```python
from build123d import *

# Parameters (mm, degrees)
SKETCH1_W                = 6.4
SKETCH1_H                = 22.2
SKETCH1_W_2              = 0.8
SKETCH1_H_2              = 2
BOSS_EXTRUDE1_DEPTH      = 13.7
BOSS_EXTRUDE2_DEPTH      = 3
SKETCH2_W                = 9
SKETCH2_H                = 2.5
CUT_EXTRUDE1_DEPTH       = 27.513015672
SKETCH2_3_W              = 2.5
SKETCH2_3_H              = 3
CUT_EXTRUDE2_DEPTH       = 0.2
CUT_EXTRUDE3_DEPTH       = 0.3
BOSS_EXTRUDE3_DEPTH      = 6.5
BOSS_EXTRUDE3_DEPTH_BACK = 6.5
SKETCH4_W                = 0.7
SKETCH4_H                = 3.8
BOSS_EXTRUDE4_DEPTH      = 4
BOSS_EXTRUDE4_DEPTH_BACK = 4
SKETCH4_3_W              = 0.3
SKETCH4_3_H              = 6.2
SKETCH7_R                = 0.25
SKETCH7_W                = 6.2
SKETCH7_H                = 1
CUT_EXTRUDE4_DEPTH       = 1


with BuildPart() as part:
    # Sketch1 → Boss-Extrude1 (new body)
    with BuildSketch(Plane(origin=(0, 0, 0), x_dir=(1, 0, 0), z_dir=(0, 1, 0))):
        with Locations((0, 4.8)):
            Rectangle(SKETCH1_W, SKETCH1_H)
        with Locations((0, 13)):
            Rectangle(SKETCH1_W_2, SKETCH1_H_2, mode=Mode.SUBTRACT)
    extrude(amount=BOSS_EXTRUDE1_DEPTH)

    # Sketch1_4 → Boss-Extrude2 (add)
    # profile 1 of 2: a face of its own
    with BuildSketch(Plane(origin=(0, 0, 0), x_dir=(1, 0, 0), z_dir=(0, 1, 0))):
        with BuildLine():
            Line((12, 3.1), (3.2, 3.1))
            Line((3.2, 3.1), (3.2, -3.1))
            Line((3.2, -3.1), (12, -3.1))
            ThreePointArc((12, -3.1), (12.707106781, -2.807106781), (13, -2.1))
            Line((13, -2.1), (13, 2.1))
            ThreePointArc((13, 2.1), (12.707106781, 2.807106781), (12, 3.1))
        make_face()
        with BuildLine():
            Line((9.5, 1.6), (10.6, 1.6))
            ThreePointArc((10.6, 1.6), (12.2, 0), (10.6, -1.6))
            Line((10.6, -1.6), (9.5, -1.6))
            ThreePointArc((9.5, -1.6), (7.9, 0), (9.5, 1.6))
        make_face(mode=Mode.SUBTRACT)
    # profile 2 of 2: a face of its own
    with BuildSketch(Plane(origin=(0, 0, 0), x_dir=(1, 0, 0), z_dir=(0, 1, 0))):
        with BuildLine():
            Line((-3.2, -3.1), (-3.2, 3.1))
            Line((-3.2, 3.1), (-12, 3.1))
            ThreePointArc((-12, 3.1), (-12.707106781, 2.807106781), (-13, 2.1))
            Line((-13, 2.1), (-13, -2.1))
            ThreePointArc((-13, -2.1), (-12.707106781, -2.807106781), (-12, -3.1))
            Line((-12, -3.1), (-3.2, -3.1))
        make_face()
        with BuildLine():
            ThreePointArc((-10.6, -1.6), (-12.2, 0), (-10.6, 1.6))
            Line((-10.6, 1.6), (-9.5, 1.6))
            ThreePointArc((-9.5, 1.6), (-7.9, 0), (-9.5, -1.6))
            Line((-9.5, -1.6), (-10.6, -1.6))
        make_face(mode=Mode.SUBTRACT)
    extrude(amount=BOSS_EXTRUDE2_DEPTH)

    # Sketch2 → Cut-Extrude1 (cut, through all)
    with BuildSketch(Plane(origin=(3.2, 0, 0), x_dir=(0, 0, -1), z_dir=(1, 0, 0))):
        with Locations((11.4, 7.95)):
            Rectangle(SKETCH2_W, SKETCH2_H)
        with Locations((11.4, 5.45)):
            Rectangle(SKETCH2_W, SKETCH2_H)
    extrude(amount=-CUT_EXTRUDE1_DEPTH, mode=Mode.SUBTRACT)

    # Sketch2_3 → Cut-Extrude2 (cut)
    with BuildSketch(Plane(origin=(3.2, 0, 0), x_dir=(0, 0, -1), z_dir=(1, 0, 0))):
        with Locations((-0.25, 8.2)):
            Rectangle(SKETCH2_3_W, SKETCH2_3_H)
    extrude(amount=-CUT_EXTRUDE2_DEPTH, mode=Mode.SUBTRACT)

    # Sketch3 → Cut-Extrude3 (cut)
    with BuildSketch(Plane.XZ):
        Polygon((-6.45, 3.1), (-3.2, 3.1), (-3.2, 6.3), (3.2, 6.3), (3.2, 3.1), (6.45, 3.1), (6.45, -3.1), (3.2, -3.1), (3.2, -15.9), (-3.2, -15.9), (-3.2, -3.1), (-6.45, -3.1), align=None)
    extrude(amount=-CUT_EXTRUDE3_DEPTH, mode=Mode.SUBTRACT)

    # Sketch4 → Boss-Extrude3 (add, two sides: drawn at the far end of the back side and taken through both)
    with BuildSketch(Plane(origin=(0, 7, 0), x_dir=(1, 0, 0), z_dir=(0, 1, 0)).offset(-BOSS_EXTRUDE3_DEPTH_BACK)):
        with Locations((2.85, -8.2)):
            Rectangle(SKETCH4_W, SKETCH4_H)
    extrude(amount=BOSS_EXTRUDE3_DEPTH + BOSS_EXTRUDE3_DEPTH_BACK)

    # Sketch4_3 → Boss-Extrude4 (add, two sides: drawn at the far end of the back side and taken through both)
    with BuildSketch(Plane(origin=(0, 7, 0), x_dir=(1, 0, 0), z_dir=(0, 1, 0)).offset(-BOSS_EXTRUDE4_DEPTH_BACK)):
        with Locations((0, -9.4)):
            Rectangle(SKETCH4_3_W, SKETCH4_3_H)
    extrude(amount=BOSS_EXTRUDE4_DEPTH + BOSS_EXTRUDE4_DEPTH_BACK)

    # Sketch7 → Cut-Extrude4 (cut)
    with BuildSketch(Plane.ZY.offset(0.15)):
        with Locations((11.824564477, 3.538657992)):
            Circle(SKETCH7_R)
        with Locations((11.824564477, 5.838657992)):
            Circle(SKETCH7_R)
        with Locations((11.824564477, 8.138657992)):
            Circle(SKETCH7_R)
        with Locations((11.824564477, 10.438657992)):
            Circle(SKETCH7_R)
        with BuildLine():
            Line((12.260846454, 3), (12.5, 3))
            Line((12.5, 3), (12.5, 3.239153546))
            ThreePointArc((12.5, 3.239153546), (12.429953548, 3.070046452), (12.260846454, 3))
        make_face()
        with Locations((9.4, 7.031126654)):
            Rectangle(SKETCH7_W, SKETCH7_H)
        with Locations((9.4, 9.376221563)):
            Rectangle(SKETCH7_W, SKETCH7_H)
        with Locations((9.4, 4.685096472)):
            Rectangle(SKETCH7_W, SKETCH7_H)
    extrude(amount=-CUT_EXTRUDE4_DEPTH, mode=Mode.SUBTRACT)


solid = part.part
```
Model file for the job. Use its own axes, mm. A direction names the side the tool comes from. Coordinates: 2 decimals unless noted, no trailing zeros. Write each loop counter-clockwise with the first axis right and the second up, starting at its lowest first coordinate (ties: lowest second). Pieces come first, ordered by that corner, then holes. Notation, with made-up numbers: (63.5, -35) - (106.5, -35) arc R24 cw to (106.5, -6) - close; hole circle Ø6 at (78, -26.5). An arc over 180 degrees is marked (long way). Use a Markdown table: item, result. Add a question column.
Item 1: Band-saw the part on B-B, the plane y = 2. Give the number of separate pieces and of enclosed holes in the cut face, and give its area (3 significant figures).
Item 2: 3-axis set-ups, long thin cutter, end or side, ignore diameter. For faces 5 (the face through (-10, 1, 1.6)), 6 (the face through (0, 0.3, -5)), 7 (the face through (0, 7, -6.9)): which of +Z, -Z, +X, -X, +Y, -Y reach the whole face in a straight line?
Item 3: Two-plate mould, pull along X, no slides. Class faces 1 (the face through (8, 1, -3.1)), 2 (the face through (0, 11, -14)), 3 (the face through (-3.2, 7, -5)), 4 (the face through (-12.2, 1.5, 0)): pulls with the +X half, pulls with the -X half, needs draft (parallel to the pull), parting line crosses it, or undercut.
Item 4: Band-saw the part on A-A, the plane z = 0. Write the cut outline in (x, y), and give its area (3 significant figures).
Item 5: Drill centre lines: line 1 along Z through (x, y) = (10.5, 0.75); line 2 along Y through (x, z) = (0, -11); line 3 along X through (y, z) = (9.5, -5.25). Where is each one in solid material? Low to high.
Item 6: Drop flat-ended pins along their axis: pin 1 (3 mm diameter, centred on y = 7.5, z = 0, fed in from +X); pin 2 (0.9 mm diameter, centred on x = -10, y = 1, fed in from -Z); pin 3 (5 mm diameter, centred on x = 10, y = 2.5, fed in from +Z). Give the stop position or say it passes through.
Item 7: Band-saw the part on D-D, the plane y = 12. Write the cut outline in (x, z).
Item 8: Band-saw the part on C-C, the plane z = -7.75. Write the cut outline in (x, y), and give its area (3 significant figures).
A:
| question | item | result |
|---|---|---|
| 1 | separate pieces | 1 |
| 1 | enclosed holes | 3 |
| 1 | area | 241 mm² |
| 2 | face 5 | +Y, -Y |
| 2 | face 6 | +Z, -Z, -Y |
| 2 | face 7 | -Z, +X, -X |
| 3 | face 1 | needs draft |
| 3 | face 2 | undercut |
| 3 | face 3 | pulls with the -X half |
| 3 | face 4 | undercut |
| 4 | outline | (-13, 0) - (-12.2, 0) - (-12.2, 3) - (-13, 3) - close; (-7.9, 0) - (-6.45, 0) - (-6.45, 0.3) - (6.45, 0.3) - (6.45, 0) - (7.9, 0) - (7.9, 3) - (3.2, 3) - (3.2, 6.7) - (3, 6.7) - (3, 9.7) - (3.2, 9.7) - (3.2, 13.7) - (-3.2, 13.7) - (-3.2, 3) - (-7.9, 3) - close; (12.2, 0) - (13, 0) - (13, 3) - (12.2, 3) - close |
| 4 | area | 116 mm² |
| 5 | line 1 | z = -3.1 to -1.6, 1.6 to 3.1 |
| 5 | line 2 | y = 0.3 to 4.2, 9.2 to 13.7 |
| 5 | line 3 | x = -3.2 to 3.2 |
| 6 | pin 1 | stops at x = 3.2 |
| 6 | pin 2 | stops at z = -3.1 |
| 6 | pin 3 | stops at z = 3.1 |
| 7 | outline | (-3.2, -15.9) - (3.2, -15.9) - (3.2, 10.1) - (2.5, 10.1) - (2.5, 6.3) - (-3.2, 6.3) - close; hole (-0.4, -14) - (0.4, -14) - (0.4, -12) - (-0.4, -12) - close |
| 8 | outline | (-3.2, 0.3) - (3.2, 0.3) - (3.2, 4.2) - (-3.2, 4.2) - close; (-3.2, 9.2) - (3.2, 9.2) - (3.2, 13.7) - (-3.2, 13.7) - close |
| 8 | area | 53.8 mm² |
